Could you check a few things on this model? Use its own coordinates, in mm. Face numbers are marked on the shaded views. Give positions to 0.01 mm unless a question says otherwise; leave off trailing zeros. Loops run counter-clockwise (first coordinate to the right, second up) from the corner with the lowest first, then second, coordinate; pieces in that order, holes last. Notation, with made-up numbers: (74, -29) - (98, -29) arc R35 cw to (98, 6) - close; hole circle Ø2 at (7, 55). An arc over 180 degrees is marked (long way). Write each question's results on one line, items separated by ' | '. Start each with the question number.
1) If we mould it in two halves opening along X, with no side actions, what happens to the marked faces 1, 2 and 3? For each: +X half, -X half, draft (parallel to the pull), parting line (faces both ways), or undercut.
2) I'm going to push flat-ended pins straight in: pin 1 (5 mm diameter, centred on x = 4.95, y = -4.95, fed in from +Z); pin 2 (1 mm diameter, centred on y = 9, z = 4, fed in from +X); pin 3 (2.5 mm diameter, centred on x = -4.95, y = 4.95, fed in from -Z). Where does each tip first touch, or does it pass through?
3) I want a section at A-A, the plane y = 1.5. Write out the boundary of the cut face in (x, z), and give its area (3 significant figures).
4) I want a section at B-B, the plane x = -10. Write out the boundary of the cut face in (y, z), and give its area (3 significant figures).
5) If I drill on probe 1 along X at (y, z) = (3.5, 3.15); probe 2 along Y at (x, z) = (-8, 3.1); probe 3 along X at (y, z) = (-4, 2.5), over which ranges is the centre line in solid material (lowest first)? Write a range as [from, to].
from build123d import *

# Parameters (mm, degrees)
SKETCH1_R           = 1.6
BOSS_EXTRUDE1_DEPTH = 4.6
CUT_EXTRUDE2_DEPTH  = 1.4


with BuildPart() as part:
    # Sketch1 → Boss-Extrude1 (new body)
    with BuildSketch(Plane.XY):
        with BuildLine():
            Line((-2.938926261, 25.327361545), (-23.179574078, 10.621670112))
            ThreePointArc((-23.179574078, 10.621670112), (-24.995930398, 8.121670112), (-24.995930398, 5.031500168))
            Line((-24.995930398, 5.031500168), (-17.264690886, -18.762808399))
            ThreePointArc((-17.264690886, -18.762808399), (-15.448334566, -21.262808399), (-12.509408305, -22.217723427))
            Line((-12.509408305, -22.217723427), (12.509408305, -22.217723427))
            ThreePointArc((12.509408305, -22.217723427), (15.448334566, -21.262808399), (17.264690886, -18.762808399))
            Line((17.264690886, -18.762808399), (24.995930398, 5.031500168))
            ThreePointArc((24.995930398, 5.031500168), (24.995930398, 8.121670112), (23.179574078, 10.621670112))
            Line((23.179574078, 10.621670112), (2.938926261, 25.327361545))
            ThreePointArc((2.938926261, 25.327361545), (0, 26.282276573), (-2.938926261, 25.327361545))
        make_face()
        with Locations((-4.949747468, 4.949747468)):
            Circle(SKETCH1_R, mode=Mode.SUBTRACT)
        with Locations((4.949747468, 4.949747468)):
            Circle(SKETCH1_R, mode=Mode.SUBTRACT)
        with Locations((4.949747468, -4.949747468)):
            Circle(SKETCH1_R, mode=Mode.SUBTRACT)
        with Locations((-4.949747468, -4.949747468)):
            Circle(SKETCH1_R, mode=Mode.SUBTRACT)
    extrude(amount=BOSS_EXTRUDE1_DEPTH)

    # Sketch3 → Cut-Extrude2 (cut)
    with BuildSketch(Plane.XY.offset(4.6)):
        with BuildLine():
            Line((-22.523183456, 5.834944354), (-14.791943944, -17.959364213))
            ThreePointArc((-14.791943944, -17.959364213), (-13.92009291, -19.159364213), (-12.509408305, -19.617723427))
            Line((-12.509408305, -19.617723427), (12.509408305, -19.617723427))
            ThreePointArc((12.509408305, -19.617723427), (13.92009291, -19.159364213), (14.791943944, -17.959364213))
            Line((14.791943944, -17.959364213), (22.523183456, 5.834944354))
            ThreePointArc((22.523183456, 5.834944354), (22.523183456, 7.318225927), (21.651332422, 8.518225927))
            Line((21.651332422, 8.518225927), (1.410684606, 23.22391736))
            ThreePointArc((1.410684606, 23.22391736), (0, 23.682276573), (-1.410684606, 23.22391736))
            Line((-1.410684606, 23.22391736), (-21.651332422, 8.518225927))
            ThreePointArc((-21.651332422, 8.518225927), (-22.523183456, 7.318225927), (-22.523183456, 5.834944354))
        make_face()
    extrude(amount=-CUT_EXTRUDE2_DEPTH, mode=Mode.SUBTRACT)


solid = part.part
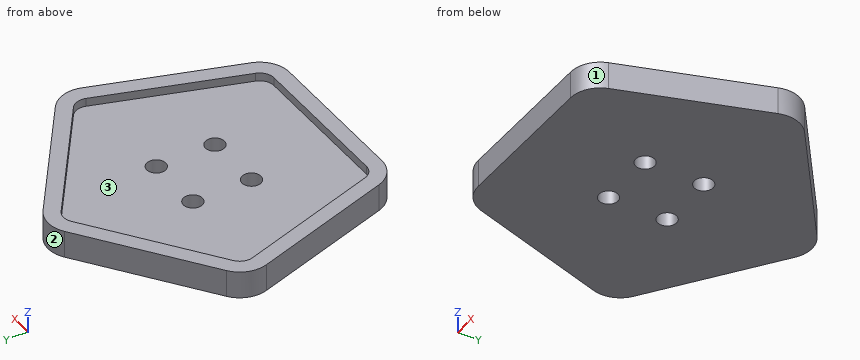
Answers:
1) face 1: +X half | face 2: parting line | face 3: undercut
2) pin 1: stops at z = 3.2 | pin 2: stops at x = 24.86 | pin 3: passes through
3) outline: (-23.85, 0) - (23.85, 0) - (23.85, 4.6) - (21.11, 4.6) - (21.11, 3.2) - (-21.11, 3.2) - (-21.11, 4.6) - (-23.85, 4.6) - close | area: 160 mm2
4) outline: (-22.22, 0) - (20.2, 0) - (20.2, 4.6) - (16.98, 4.6) - (16.98, 3.2) - (-19.62, 3.2) - (-19.62, 4.6) - (-22.22, 4.6) - close | area: 144 mm2
5) probe 1: x = [-24.5, -5.63], [-4.27, 4.27], [5.63, 24.5] | probe 2: y = [-22.22, 21.65] | probe 3: x = [-22.06, -6.24], [-3.66, 3.66], [6.24, 22.06]
